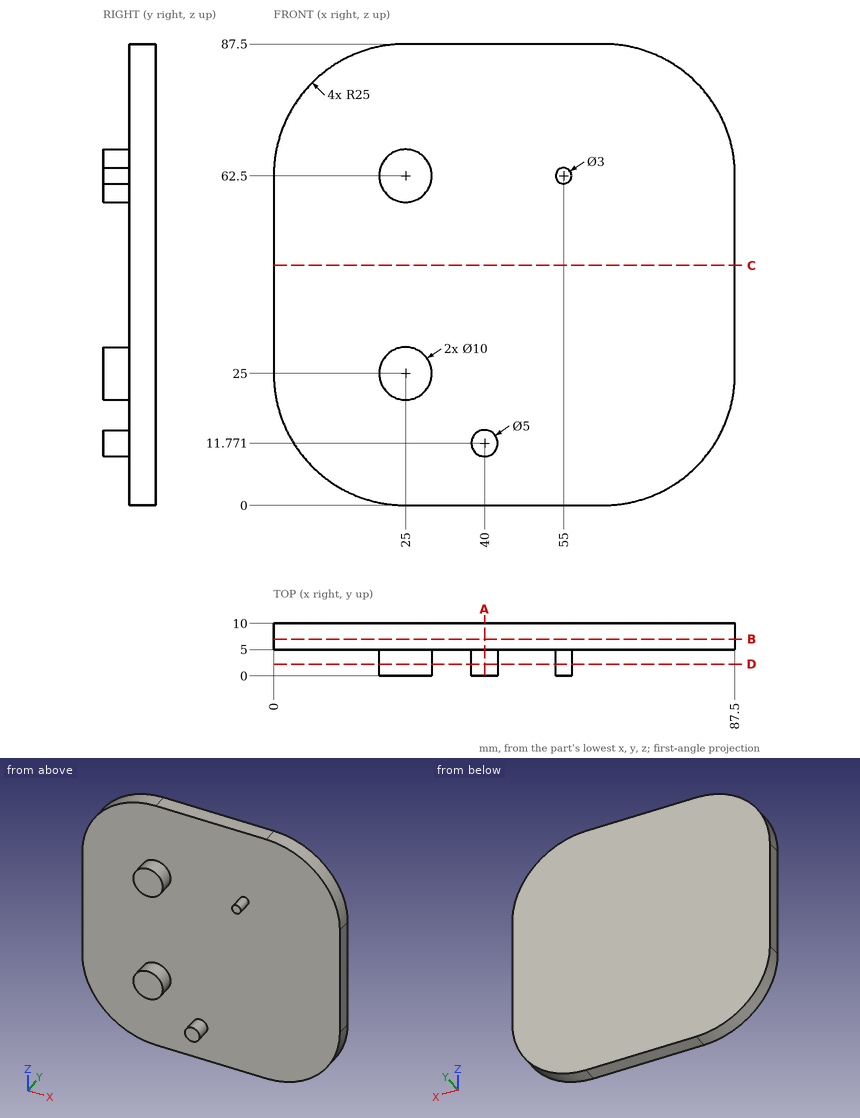
Geometry check sheet. Reference: drawing and pictorial views, mm from the part's lowest x, y, z. Coordinates: 2 decimals unless noted, no trailing zeros. Write each loop counter-clockwise with the first axis right and the second up, starting at its lowest first coordinate (ties: lowest second). Pieces come first, ordered by that corner, then holes. Notation, with made-up numbers: (5.25, -12.75) -> (54.25, -12.75) arc R15 cw to (54.25, -3.75) -> close; hole circle Ø8 at (74, 52). An arc over 180 degrees is marked (long way). Use a Markdown table: item, result.
1. Scan lines: line 1 along Y through (x, z) = (11, 57.5); line 2 along Z through (x, y) = (26.5, 1.25); line 3 along Z through (x, y) = (18, 7.25). Record each from-to range of solid material in increasing order.
Reported:
| item | result |
|---|---|
| line 1 | y = 5 to 10 |
| line 2 | z = 20.23 to 29.77, 57.73 to 67.27 |
| line 3 | z = 1 to 86.5 |
2. Go/stop test with flat-tipped pins: pin 1 Ø5 at (x, y) = (42.5, 3.5) entering from -Z; pin 2 Ø5 at (x, y) = (24.5, 2) entering from -Z. Record where each tip stops, or that it passes through.
Reported:
| item | result |
|---|---|
| pin 1 | stops at z = 0 |
| pin 2 | stops at z = 20 |
3. Sectioned sample at D-D (y = 2.25). Enter the section's corners in (x, z), plus the area to 3 significant figures.
Reported:
| item | result |
|---|---|
| outline | circle Ø10 at (25, 25); circle Ø10 at (25, 62.5); circle Ø5 at (40, 11.77); circle Ø3 at (55, 62.5) |
| area | 184 mm2 |
4. Sectioned sample at B-B (y = 7). Enter the section's corners in (x, z).
Reported:
| item | result |
|---|---|
| outline | (0, 25) arc R25 ccw to (25, 0) -> (62.5, 0) arc R25 ccw to (87.5, 25) -> (87.5, 62.5) arc R25 ccw to (62.5, 87.5) -> (25, 87.5) arc R25 ccw to (0, 62.5) -> close |
5. Sectioned sample at A-A (x = 40). Enter the section's corners in (y, z).
Reported:
| item | result |
|---|---|
| outline | (0, 9.27) -> (5, 9.27) -> (5, 0) -> (10, 0) -> (10, 87.5) -> (5, 87.5) -> (5, 14.27) -> (0, 14.27) -> close |
6. Sectioned sample at C-C (z = 45.5). Enter the section's corners in (x, y).
Reported:
| item | result |
|---|---|
| outline | (0, 5) -> (87.5, 5) -> (87.5, 10) -> (0, 10) -> close |
